```python
from build123d import *

# Parameters (mm, degrees)
CROQUIS2_R              = 50
SALIENTE_EXTRUIR1_DEPTH = 12
CROQUIS2_3_R            = 11
CORTAR_EXTRUIR1_DEPTH   = 2
CROQUIS2_6_R            = 8
CORTAR_EXTRUIR4_DEPTH   = 2
TALADRO_ROSCADO_G1_81_D = 8.8
CORTAR_EXTRUIR3_DEPTH   = 2
MATRIZC1_COUNT          = 5
CROQUIS7_W              = 3.7
CROQUIS7_H              = 4.2
TALADRO_ROSCADO_M51_D   = 4.2
MATRIZC2_COUNT          = 6


with BuildPart() as part:
    # Croquis2 → Saliente-Extruir1 (new body)
    with BuildSketch(Plane(origin=(0, 0, 0), x_dir=(1, 0, 0), z_dir=(0, 1, 0))):
        Circle(CROQUIS2_R)
    extrude(amount=-SALIENTE_EXTRUIR1_DEPTH)

    # Croquis2<3> → Cortar-Extruir1 (cut)
    with BuildSketch(Plane(origin=(0, 0, 0), x_dir=(1, 0, 0), z_dir=(0, 1, 0))):
        with Locations((0, 20)):
            Circle(CROQUIS2_3_R)
    cortar_extruir1 = extrude(amount=-CORTAR_EXTRUIR1_DEPTH, mode=Mode.SUBTRACT)

    # Croquis2<6> → Cortar-Extruir4 (cut)
    with BuildSketch(Plane(origin=(0, 0, 0), x_dir=(1, 0, 0), z_dir=(0, 1, 0))):
        Circle(CROQUIS2_6_R)
    extrude(amount=-CORTAR_EXTRUIR4_DEPTH, mode=Mode.SUBTRACT)

    # Taladro roscado G1/81 (through all)
    with Locations(Plane(origin=(0, -12, 0), x_dir=(-1, 0, 0), z_dir=(0, -1, 0))):
        with Locations((0, 0)):
            Hole(TALADRO_ROSCADO_G1_81_D / 2)

    # Croquis6 → Cortar-Extruir3 (cut)
    with BuildSketch(Plane(origin=(0, 0, 0), x_dir=(1, 0, 0), z_dir=(0, 1, 0))):
        with BuildLine():
            Line((1.5, 20), (1.5, 0))
            ThreePointArc((1.5, 0), (0, -1.5), (-1.5, 0))
            Line((-1.5, 0), (-1.5, 20))
            ThreePointArc((-1.5, 20), (0, 21.5), (1.5, 20))
        make_face()
    cortar_extruir3 = extrude(amount=-CORTAR_EXTRUIR3_DEPTH, mode=Mode.SUBTRACT)

    # MatrizC1: Cortar-Extruir1, Cortar-Extruir3 ×5 about axis
    matrizc1_axis = Axis((0, 0, 0), (0, 1, 0))
    for i in range(1, MATRIZC1_COUNT):
        add(cortar_extruir1.rotate(matrizc1_axis, i * 360 / MATRIZC1_COUNT), mode=Mode.SUBTRACT)
        add(cortar_extruir3.rotate(matrizc1_axis, i * 360 / MATRIZC1_COUNT), mode=Mode.SUBTRACT)

    # Croquis7 → Cortar-Revolución1 (revolve, cut)
    with BuildSketch(Plane(origin=(0, 0, 0), x_dir=(0, 0, -1), z_dir=(1, 0, 0))):
        with Locations((35.285, 0)):
            Rectangle(CROQUIS7_W, CROQUIS7_H)
    revolve(axis=Axis((0, 0, 0), (0, -1, 0)), mode=Mode.SUBTRACT)

    # Taladro roscado M51 (through all)
    with Locations(Plane(origin=(0, 0, 0), x_dir=(1, 0, 0), z_dir=(0, 1, 0))):
        with Locations((0, 44)):
            taladro_roscado_m51 = Hole(TALADRO_ROSCADO_M51_D / 2)

    # MatrizC2: Taladro roscado M51 ×6 about axis
    matrizc2_axis = Axis((0, 0, 0), (0, 1, 0))
    for i in range(1, MATRIZC2_COUNT):
        add(taladro_roscado_m51.rotate(matrizc2_axis, i * 360 / MATRIZC2_COUNT), mode=Mode.SUBTRACT)


solid = part.part
```
Here's how the part is built. I have some questions about the finished solid (model axes, mm). A direction names the side the tool comes from. Give positions to 0.01 mm unless a question says otherwise; leave off trailing zeros. Write each loop counter-clockwise with the first axis right and the second up, starting at its lowest first coordinate (ties: lowest second). Pieces come first, ordered by that corner, then holes.
(1) Imagine slicing it at C-C, the plane z = 22. Write out the boundary of the cut face in (x, y), and give its area (3 significant figures).
Output values:
outline: (-44.9, -12) - (-40.21, -12) - (-40.21, 0) - (-44.9, 0) - close; (-36.01, -12) - (36.01, -12) - (36.01, 0) - (29.92, 0) - (29.92, -2.1) - (25.18, -2.1) - (25.18, 0) - (21.09, 0) - (21.09, -2) - (2.42, -2) - (2.42, 0) - (-2.42, 0) - (-2.42, -2) - (-21.09, -2) - (-21.09, 0) - (-25.18, 0) - (-25.18, -2.1) - (-29.92, -2.1) - (-29.92, 0) - (-36.01, 0) - close; (40.21, -12) - (44.9, -12) - (44.9, 0) - (40.21, 0) - close
area: 882 mm2
(2) Imagine slicing it at B-B, the plane y = -6.5. Write out the boundary of the cut face in (x, z), and give its area (3 significant figures).
Output values:
outline: circle Ø100 at (0, 0); hole circle Ø4.2 at (-38.11, -22); hole circle Ø4.2 at (-38.11, 22); hole circle Ø8.8 at (0, 0); hole circle Ø4.2 at (0, -44); hole circle Ø4.2 at (0, 44); hole circle Ø4.2 at (38.11, -22); hole circle Ø4.2 at (38.11, 22)
area: 7,710 mm2
(3) Will these pins go through, and if not, where does the flat tip stop? pin 1 (3 mm diameter, centred on x = -17.5, y = -10.5, fed in from -Z); pin 2 (5 mm diameter, centred on y = -10, z = 18, fed in from -X); pin 3 (1 mm diameter, centred on y = -1, z = -8.5, fed in from -X).
Output values:
pin 1: stops at z = -47.37
pin 2: stops at x = -47.54
pin 3: stops at x = -49.36
(4) Thinking about a two-plate mould opening in Z: for faces 3 (the face through (-8, 0, 37)), 4 (the face through (-18.59, -0.99, 24.8)), 5 (the face through (-4, -2, 6)), which applies, pulls with the +Z half, pulls with the -Z half, needs draft (parallel to the pull), parting line crosses it, or undercut?
Output values:
face 3: needs draft
face 4: undercut
face 5: undercut
(5) Imagine slicing it at D-D, the plane x = 32. Write out the boundary of the cut face in (y, z).
Output values:
outline: (-12, -38.42) - (0, -38.42) - (0, -18.84) - (-2.1, -18.84) - (-2.1, -9.69) - (0, -9.69) - (0, 9.69) - (-2.1, 9.69) - (-2.1, 18.84) - (0, 18.84) - (0, 38.42) - (-12, 38.42) - close
(6) On a 3-axis mill with a long thin cutter (end or side, diameter ignored), from which of +Z, -Z, +X, -X, +Y, -Y can I reach the whole of each face in a straight line? I mean faces 1 (the face through (4.742, -0.986, -6.443)), 2 (the face through (-36.56, -6.08, 20.58)). Say none if no direction works.
Output values:
face 1: +Y
face 2: +Y, -Y
(7) Imagine slicing it at A-A, the plane z = 44. Write out the boundary of the cut face in (x, y).
Output values:
outline: (-23.75, -12) - (-2.1, -12) - (-2.1, 0) - (-23.75, 0) - close; (2.1, -12) - (23.75, -12) - (23.75, 0) - (2.1, 0) - close
(8) If I drill on L1, parallel to Z at x = 0, y = -5.75; L2, parallel to X at y = -0.6, z = 0 (1 decimal); L3, parallel to X at y = -0.25, z = -19.5, over which ranges is the centre line in solid material (lowest first)?
Output values:
L1: z = -50 to -46.1, -41.9 to -4.4, 4.4 to 41.9, 46.1 to 50
L2: x = -50 to -37.1, -33.4 to -28.1, -9.9 to -8, 8 to 9.9, 28.1 to 33.4, 37.1 to 50
L3: x = -46.04 to -31.6, -27.16 to -10.99, 10.99 to 27.16, 31.6 to 46.04
